CAD build for the part. Positions are in the model's coordinates, mm. A direction names the side the tool comes from. Give positions to 0.01 mm unless a question says otherwise; leave off trailing zeros. Write each loop counter-clockwise with the first axis right and the second up, starting at its lowest first coordinate (ties: lowest second). Pieces come first, ordered by that corner, then holes. Notation, with made-up numbers: (47.5, 80) - (84.5, 80) arc R17 cw to (84.5, 97) - close; hole circle Ø2 at (17, 20). An arc over 180 degrees is marked (long way). Answer as a JSON object with one key per item and string values.
Autodesk Inventor part; units mm, degrees
ref_plane "YZ Plane" through (0, 0, 0) normal (1, 0, 0) x (0, 1, 0)
ref_plane "XZ Plane" through (0, 0, 0) normal (0, 1, 0) x (-1, 0, 0)
ref_plane "XY Plane" through (0, 0, 0) normal (0, 0, 1) x (1, 0, 0)
sketch "スケッチ1" plane through (0, 0, 0) normal (0, 0, 1) x (1, 0, 0)
  line L0 (369, -217.5) -> (-369, -217.5)
  line L1 (-369, -217.5) -> (-369, 217.5)
  line L2 (-369, 217.5) -> (369, 217.5)
  line L3 (369, 217.5) -> (369, -217.5)
  line L4 (369, -217.5) -> (-369, 217.5) construction
  line L5 (-369, -217.5) -> (369, 217.5) construction
  point P0 (0, 0)
  dimension "d0" = 738
  dimension "d1" = 435
extrude "押し出し1" add sketch "スケッチ1" along normal blind 59
sketch "スケッチ2" plane through (369, -217.5, 0) normal (1, 0, 0) x (0, 0, -1)
  line L0 (0, 435) -> (-59, 435)
  line L1 (-42.8, 435) -> (0, 435)
  line L2 (0, 435) -> (0, 235)
  line L3 (0, 235) -> (-42.8, 235)
  line L4 (-42.8, 235) -> (-42.8, 435)
  line L5 (-59, 0) -> (-59, 435)
  point P0 (0, 217.5)
  dimension "d4" = 16.2
  dimension "d5" = 200
extrude "押し出し2" cut sketch "スケッチ2" against normal through all
chamfer "面取り1" distance 20 angle 45 1 edges at (0, 17.5, 42.8)
fillet "フィレット1" radius 5 3 edges at (0, 37.5, 42.8) (0, 17.5, 22.8) (0, 17.5, 0)
properties part number "Display_A"
Item 1: Which spindle directions (+Z, -Z, +X, -X, +Y, -Y) get a long thin tool onto all of the face, cutting with end or side? Do faces 1 (the flat face through (5, 127, 42.8)), 2 (the flat face through (-5, -101, 0)). Say none if no direction does.
Entries:
{"face 1": "-Z, +X, -X, +Y", "face 2": "-Z, +X, -X, +Y, -Y"}
Item 2: Cut at B-B (y = 70.5). Give the cut face in (x, z), and give its area (3 significant figures).
Entries:
{"outline": "(-369, 42.8) - (369, 42.8) - (369, 59) - (-369, 59) - close", "area": "12,000 mm2"}
Item 3: Mould opens along X. For faces 3 (the flat face through (369, -45, 36)), 4 (the flat face through (-369, -51, 36)), 5 (the flat face through (-5, 3, 59)) say: +X half, -X half, draft (parallel to the pull), parting line (faces both ways), or undercut.
Entries:
{"face 3": "+X half", "face 4": "-X half", "face 5": "draft"}
Item 4: Probe line 1 (Z direction, x = -60, y = 121.5); line 2 (Y direction, x = -41, z = 21); line 3 (Y direction, x = 334, z = 41.5). List the from-to ranges inside material, lowest first. Write a range as from..to.
Entries:
{"line 1": "42.8..59", "line 2": "-217.5..17.51", "line 3": "-217.5..36.21"}
Item 5: Cut at A-A (x = -206). Give the cut face in (y, z), and give its area (3 significant figures).
Entries:
{"outline": "(-217.5, 0) - (12.5, 0) arc R5 ccw to (17.5, 5) - (17.5, 20.73) arc R5 cw to (18.96, 24.26) - (36.04, 41.34) arc R5 cw to (39.57, 42.8) - (217.5, 42.8) - (217.5, 59) - (-217.5, 59) - close", "area": "17,300 mm2"}
Item 6: Flat gauge pin, fed straight in: P1, Ø8, axis at x = -73.5, z = 12, coming from the +Y side. Where does the tip first touch, or does it go through?
Entries:
{"P1": "y = 17.5"}
